Autodesk Inventor part; units mm, degrees
ref_plane "YZ Plane" through (0, 0, 0) normal (1, 0, 0) x (0, 1, 0)
ref_plane "XZ Plane" through (0, 0, 0) normal (0, 1, 0) x (-1, 0, 0)
ref_plane "XY Plane" through (0, 0, 0) normal (0, 0, 1) x (1, 0, 0)
sketch "Sketch1" plane through (0, 0, 0) normal (0, 1, 0) x (-1, 0, 0)
  line L0 (0, 0) -> (35, 0)
  line L1 (35, 0) -> (35, -57)
  line L2 (35, -57) -> (0, -57)
  line L3 (0, -57) -> (0, 0)
  dimension "d0" = 35
  dimension "d1" = 57
extrude "Extrusion1" add sketch "Sketch1" along normal blind 1
sketch "Sketch2" plane through (0, 1, 0) normal (0, 1, 0) x (1, 0, 0)
  line L0 (-35, 0) -> (0, 0)
  line L1 (0, 57) -> (-35, 57)
  line L2 (0, 0) -> (-1, 0)
  line L3 (-1, 0) -> (-1, 57)
  line L4 (-1, 57) -> (0, 57)
  line L5 (0, 57) -> (0, 0)
  line L6 (-31, 0) -> (-30, 0)
  line L7 (-30, 0) -> (-30, 7)
  line L8 (-30, 7) -> (-31, 7)
  line L9 (-31, 7) -> (-31, 0)
  line L10 (-31, 57) -> (-30, 57)
  line L11 (-30, 57) -> (-30, 50)
  line L12 (-30, 50) -> (-31, 50)
  line L13 (-31, 50) -> (-31, 57)
  dimension "d4" = 1
  dimension "d5" = 31
  dimension "d6" = 1
  dimension "d7" = 7
  dimension "d8" = 7
extrude "Extrusion2" add sketch "Sketch2" along normal blind 24
sketch "Sketch3" plane through (-30, 1, 0) normal (1, 0, 0) x (0, 0, -1)
  line L0 (0, 24) -> (7, 24)
  line L1 (3.5, 24) -> (3.5, 19)
  line L2 (3.5, 19) -> (3.5, 9)
  line L3 (50, 24) -> (57, 24)
  line L4 (53.5, 24) -> (53.5, 19)
  line L5 (53.5, 19) -> (53.5, 9)
  circle A0 centre (3.5, 19) radius 1
  circle A1 centre (3.5, 9) radius 1
  circle A2 centre (53.5, 19) radius 1
  circle A3 centre (53.5, 9) radius 1
  point P0 (0, -1)
  dimension "d11" = 5
  dimension "d12" = 10
  dimension "d13" = 5
  dimension "d14" = 10
  dimension "d15" = 2
  dimension "d16" = 2
  dimension "d17" = 2
  dimension "d18" = 2
extrude "Extrusion3" cut sketch "Sketch3" against normal blind 24
properties part number "elbow servo plate"
Geometry check sheet. Reference: the model listing, model coordinates, mm. A direction names the side the tool comes from. Round coordinates to 2 decimals unless told otherwise and drop trailing zeros. Order: outer loops, then holes, each group sorted by start corner. A loop starts at its lowest first (then second) coordinate and runs counter-clockwise, first axis right, second up. Notation, with made-up numbers: (-11.75, 41) -> (37.25, 41) arc R11 ccw to (37.25, 54) -> close; hole circle Ø6 at (65, 39). An arc over 180 degrees is marked (long way). Return JSON: item names as keys, results as strings. Group by question number.
Q1. Section check C-C, the plane y = 20. Record the boundary of the cut face in (x, z).
Q2. Section check B-B, the plane y = 6.25. Record the boundary of the cut face in (x, z).
Q3. Release check for a two-part mould opening along Y. For faces 6 (the flat face through (-30, 13, -54)), 7 (the cylindrical face through (-30.49, 10.99, -3.37)), 8 (the cylindrical face through (-30.493, 19.024, -3.283)), 9 (the flat face through (-17, 0, -28)) record: released by +Y, released by -Y, zero draft, split by the parting line, or undercut.
Q4. Material ranges on probe 1 along Y at (x, z) = (-30.6, -53.5); probe 2 along Z at (x, y) = (-30.55, 10); probe 3 along X at (y, z) = (15.5, -5), recorded low to high. Write a range as from..to.
Q5. Tool access check on faces 1 (the flat face through (0, 12, -29)), 2 (the flat face through (-30, 13, -3)), 3 (the flat face through (-31, 13, -4)), 4 (the cylindrical face through (-30.493, 10.676, -52.763)), 5 (the flat face through (-16.1, 0.4, 0)). Record the directions out of +Z, -Z, +X, -X, +Y, -Y that give a thin tool (end or side, any length) a straight path to the whole face; none if there is none.
Q6. Section check A-A, the plane z = -3.5. Record the boundary of the cut face in (x, y).
Q7. Section check D-D, the plane z = -51. Record the boundary of the cut face in (x, y).
Q8. Gauge pin test, flat ends, axial feed: pin 1 (1.8 mm diameter, centred on y = 10, z = -3.5, fed in from -X); pin 2 (3.5 mm diameter, centred on y = 12.5, z = -4.5, fed in from -X); pin 3 (10 mm diameter, centred on x = -21.5, z = -16.5, fed in from +Y). Record the tip position at first contact, or that the pin passes through.
Numbers:
{
 "1": {"outline": "(-31, -57) -> (-30, -57) -> (-30, -54.5) -> (-31, -54.5) -> close; (-31, -52.5) -> (-30, -52.5) -> (-30, -50) -> (-31, -50) -> close; (-31, -7) -> (-30, -7) -> (-30, -4.5) -> (-31, -4.5) -> close; (-31, -2.5) -> (-30, -2.5) -> (-30, 0) -> (-31, 0) -> close; (-1, -57) -> (0, -57) -> (0, 0) -> (-1, 0) -> close"},
 "2": {"outline": "(-31, -57) -> (-30, -57) -> (-30, -50) -> (-31, -50) -> close; (-31, -7) -> (-30, -7) -> (-30, 0) -> (-31, 0) -> close; (-1, -57) -> (0, -57) -> (0, 0) -> (-1, 0) -> close"},
 "3": {"face 6": "zero draft", "face 7": "undercut", "face 8": "undercut", "face 9": "released by -Y"},
 "4": {"probe 1": "0..9, 11..19, 21..25", "probe 2": "-57..-54.5, -52.5..-50, -7..-4.5, -2.5..0", "probe 3": "-31..-30, -1..0"},
 "5": {"face 1": "+Z, -Z, +X, +Y, -Y", "face 2": "+Z, -Z, +Y", "face 3": "+Z, -Z, -X, +Y", "face 4": "-X", "face 5": "+Z, +X, -X, +Y, -Y"},
 "6": {"outline": "(-35, 0) -> (0, 0) -> (0, 25) -> (-1, 25) -> (-1, 1) -> (-30, 1) -> (-30, 9) -> (-31, 9) -> (-31, 1) -> (-35, 1) -> close; (-31, 11) -> (-30, 11) -> (-30, 19) -> (-31, 19) -> close; (-31, 21) -> (-30, 21) -> (-30, 25) -> (-31, 25) -> close"},
 "7": {"outline": "(-35, 0) -> (0, 0) -> (0, 25) -> (-1, 25) -> (-1, 1) -> (-30, 1) -> (-30, 25) -> (-31, 25) -> (-31, 1) -> (-35, 1) -> close"},
 "8": {"pin 1": "x = -1", "pin 2": "x = -31", "pin 3": "y = 1"}
}
